```python
from build123d import *

# Parameters (mm, degrees)
F1_DEPTH = 127
F3_DEPTH = 38.1
F4_DEPTH = 19.05


# Not quite as in the source:
# - a pattern or mirror of a feature is missing from the dataset's text; its kind, count and spacing are read off the source's solid


with BuildPart() as f1:
    # F0 (on Front) → F1 (new body, symmetric)
    with BuildSketch(Plane.XZ):
        Polygon((0, 254), (0, 0), (254, 0), (254, 38.1), (177.8, 38.1), (38.1, 38.1), (38.1, 133.35), (38.1, 228.6), align=None)
    extrude(amount=F1_DEPTH, both=True)

    # F2 (on face) → F3 (join)
    with BuildSketch(Plane.XZ.offset(127)):
        Polygon((254, 38.1), (38.1, 139.7), (38.1, 38.1), align=None)
    f3 = extrude(amount=-F3_DEPTH)

    # F3_copies: F3 across plane
    add(f3.mirror(Plane.ZX))

    # F0 (on Front) → F4 (join, symmetric)
    with BuildSketch(Plane.XZ):
        Polygon((0, 254), (0, 0), (254, 0), (254, 38.1), (177.8, 38.1), (38.1, 38.1), (38.1, 133.35), (38.1, 228.6), align=None)
        Polygon((101.6, 133.35), (38.1, 133.35), (38.1, 38.1), (177.8, 38.1), align=None)
    extrude(amount=F4_DEPTH, both=True)


solid = f1.part
```
For this review, take the finished solid that the model builds, in its own axes (mm). A direction names the side the tool comes from. Coordinates: 2 decimals unless noted, no trailing zeros. Write each loop counter-clockwise with the first axis right and the second up, starting at its lowest first coordinate (ties: lowest second). Pieces come first, ordered by that corner, then holes. Notation, with made-up numbers: (-24, -32.75) - (-17, -32.75) arc R24 ccw to (-17, 0.25) - close; hole circle Ø10 at (59.5, 58.5). An arc over 180 degrees is marked (long way). Answer in a Markdown table with one row per item. Add a question column.
Q1. We need section A-A, the plane z = 62.5. State the section outline as (x, y) points, and give its area (3 significant figures).
Q2. For probe 1 along Y at (x, z) = (119.5, 69.5); probe 2 along Z at (x, y) = (129, 76.5), list the stretches that pass through material, from the lowest coordinate up.
Q3. We need section D-D, the plane y = -53.5. State the section outline as (x, z) points, and give its area (3 significant figures).
Q4. We need section C-C, the plane x = 187.5. State the section outline as (y, z) points, and give its area (3 significant figures).
Q5. Draft analysis for pull direction Y (two halves, no side actions). For faces 1 (the flat face through (97, 127, 72)), 2 (the flat face through (97, -88.9, 67)), 3 (the flat face through (147.56, 108.22, 88.19)), 4 (the flat face through (97, 88.9, 67)), state which applies: +Y half, -Y half, draft (parallel to the pull), parting line (faces both ways), or undercut.
Q6. For P1, Ø19, axis at x = 85, y = -9.5, coming from the +Z side; P2, Ø5, axis at y = -29, z = 207, coming from the +X side; P3, Ø3, axis at x = 48, y = 74.5, coming from the +Z side, all flat-tipped, find the tip position at first contact; note any pin that passes through.
Q7. We need section B-B, the plane y = -13. State the section outline as (x, z) points, and give its area (3 significant figures).
Q8. Tool access review of faces 5 (the flat face through (147.56, -108.22, 88.19)), 6 (the flat face through (140.2, -0.3, 85.1)), 7 (the flat face through (125, -2, 0)): name each direction out of +Z, -Z, +X, -X, +Y, -Y from which nothing blocks a thin tool from reaching the whole face with its end or side.
Answer list:
| question | item | result |
|---|---|---|
| 1 | outline | (0, -127) - (202.15, -127) - (202.15, -88.9) - (38.1, -88.9) - (38.1, -19.05) - (158.28, -19.05) - (158.28, 19.05) - (38.1, 19.05) - (38.1, 88.9) - (202.15, 88.9) - (202.15, 127) - (0, 127) - close |
| 1 | area | 26,800 mm2 |
| 2 | probe 1 | y = -127 to -88.9, -19.05 to 19.05, 88.9 to 127 |
| 2 | probe 2 | z = 0 to 38.1 |
| 3 | outline | (0, 0) - (254, 0) - (254, 38.1) - (38.1, 38.1) - (38.1, 228.6) - (0, 254) - close |
| 3 | area | 17,400 mm2 |
| 4 | outline | (-127, 0) - (127, 0) - (127, 69.39) - (88.9, 69.39) - (88.9, 38.1) - (-88.9, 38.1) - (-88.9, 69.39) - (-127, 69.39) - close |
| 4 | area | 12,100 mm2 |
| 5 | face 1 | +Y half |
| 5 | face 2 | undercut |
| 5 | face 3 | draft |
| 5 | face 4 | undercut |
| 6 | P1 | stops at z = 133.35 |
| 6 | P2 | stops at x = 38.1 |
| 6 | P3 | stops at z = 38.1 |
| 7 | outline | (0, 0) - (254, 0) - (254, 38.1) - (177.8, 38.1) - (101.6, 133.35) - (38.1, 133.35) - (38.1, 228.6) - (0, 254) - close |
| 7 | area | 27,100 mm2 |
| 8 | face 5 | +Z, +X, -Y |
| 8 | face 6 | +Z, +X |
| 8 | face 7 | -Z, +X, -X, +Y, -Y |
